Model file for the job. Use its own axes, mm. Coordinates: 2 decimals unless noted, no trailing zeros. Loops run counter-clockwise (first coordinate to the right, second up) from the corner with the lowest first, then second, coordinate; pieces in that order, holes last. Notation, with made-up numbers: M 79,45 L 100,45 A22 cw 100,76 Z; hole C -36,57.25 d11. An arc over 180 degrees is marked long. Write item = value, one per line. Start each with the question number.
from build123d import *

# Parameters (mm, degrees)
BOSS_EXTRUDE2_DEPTH      = 3
FILLET3_R                = 10
FILLET3_OF_MIRROR3_R     = 10
BOSS_EXTRUDE3_START      = -3
BOSS_EXTRUDE3_DEPTH      = 3
F_2_0_2_DIAMETER_HOLE1_D = 2


with BuildPart() as part:
    # Sketch2 → Boss-Extrude2 (new body)
    with BuildSketch(Plane(origin=(0, 0, 0), x_dir=(1, 0, 0), z_dir=(0, 1, 0))):
        with BuildLine():
            ThreePointArc((0, 117.185905081), (5, 117.120320028), (9.996559473, 116.923609999))
            ThreePointArc((9.996559473, 116.923609999), (7.163202874, 124.163621369), (0, 127.185905081))
            Line((0, 127.185905081), (0, 117.185905081))
        make_face()
        with BuildLine():
            Line((75, 92.603329386), (75, 4.814094919))
            ThreePointArc((75, 4.814094919), (82.067539985, 0.118365096), (86.763269807, 7.185905081))
            Line((86.763269807, 7.185905081), (85, 17.185905081))
            Line((85, 17.185905081), (85, 97.185905081))
            ThreePointArc((85, 97.185905081), (43.660622991, 112.118552795), (0, 117.185905081))
            Line((0, 117.185905081), (0, 109.185905081))
            ThreePointArc((0, 109.185905081), (38.343884954, 104.711356725), (75, 92.603329386))
        make_face()
    boss_extrude2 = extrude(amount=BOSS_EXTRUDE2_DEPTH)

    # Fillet3
    fillet3_edges = [part.edges().sort_by_distance(p)[0] for p in [
        (9.996559473, 1.5, -116.923609999),
        (85, 1.5, -97.185905081),
    ]]
    fillet(fillet3_edges, radius=FILLET3_R)

    # Mirror3: Boss-Extrude2 across plane
    add(boss_extrude2.mirror(Plane(origin=(0, 3, 0), x_dir=(0, 0, 1), z_dir=(1, 0, 0))))

    # Fillet3 of Mirror3
    fillet3_of_mirror3_edges = [part.edges().sort_by_distance(p)[0] for p in [
        (-9.996559473, 1.5, -116.923609999),
        (-85, 1.5, -97.185905081),
    ]]
    fillet(fillet3_of_mirror3_edges, radius=FILLET3_OF_MIRROR3_R)

    # Sketch4 → Boss-Extrude3 (add)
    with BuildSketch(Plane(origin=(0, 3, 0), x_dir=(1, 0, 0), z_dir=(0, 1, 0)).offset(BOSS_EXTRUDE3_START)):
        with BuildLine():
            Line((0, 109.185905081), (0, 106.185905081))
            ThreePointArc((0, 106.185905081), (2.927170094, 106.948379402), (5.110376179, 109.042013335))
            ThreePointArc((5.110376179, 109.042013335), (2.555670493, 109.131091975), (0, 109.185905081))
        make_face()
        with BuildLine():
            ThreePointArc((75, 92.603329386), (73.004956974, 93.481711721), (71, 94.337223109))
            ThreePointArc((71, 94.337223109), (72.171572875, 91.508795985), (75, 90.337223109))
            Line((75, 90.337223109), (75, 92.603329386))
        make_face()
        with BuildLine():
            Line((75, 73.103329386), (75, 82.103329386))
            ThreePointArc((75, 82.103329386), (70.5, 77.603329386), (75, 73.103329386))
        make_face()
    boss_extrude3 = extrude(amount=BOSS_EXTRUDE3_DEPTH)

    # Mirror4: Boss-Extrude3 across plane
    add(boss_extrude3.mirror(Plane(origin=(0, 0, 0), x_dir=(0, 0, 1), z_dir=(1, 0, 0))))

    # Ø2.0 (2) Diameter Hole1 (through all)
    with Locations(Plane(origin=(2.555188089, 3, -110.613959208), x_dir=(0, 0, 1), z_dir=(0, 1, 0))):
        with Locations((0, 0), (16.276736099, 72.444811911), (33.010629822, 72.444811911)):
            f_2_0_2_diameter_hole1 = Hole(F_2_0_2_DIAMETER_HOLE1_D / 2)

    # Mirror5: Ø2.0 (2) Diameter Hole1 across plane
    add(f_2_0_2_diameter_hole1.mirror(Plane(origin=(0, 0, 0), x_dir=(0, 0, 1), z_dir=(1, 0, 0))), mode=Mode.SUBTRACT)


solid = part.part
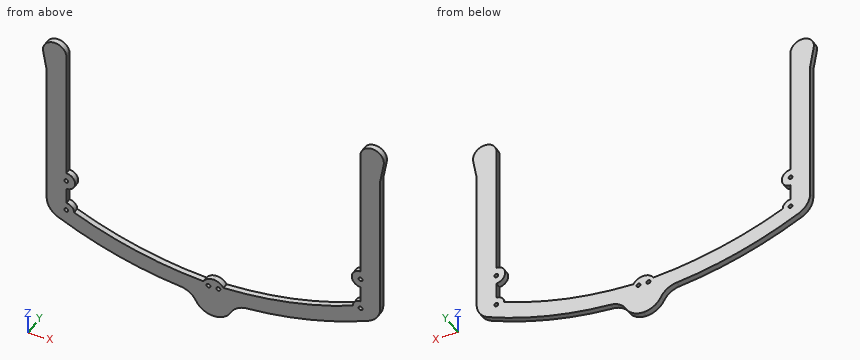
Item 1: Pin check, flat tips, straight feed: pin 1 Ø1.5 at (y, z) = (1, -85) entering from -X; pin 2 Ø1.5 at (y, z) = (1, -84.5) entering from +X; pin 3 Ø1.2 at (x, z) = (-75, -77.6) entering from +Y; pin 4 Ø1.5 at (x, y) = (-31.5, 2) entering from +Z. Stop position of each tip, or through.
Item 2: Cut at B-B (x = -62). Give the cut face in (y, z), plus the area to 3 significant figures.
Item 3: Cut at D-D (x = 36). Give the cut face in (y, z), plus the area to 3 significant figures.
Item 4: Probe L1, parallel to X at y = 0.95, z = -52; L2, parallel to X at y = 2.15, z = -5.5; L3, parallel to Z at x = 72.5, y = 0.2. List the from-to ranges inside material, lowest first.
Item 5: Cut at C-C (y = 2.25). Give the number of separate pieces and of enclosed holes in the cut face, plus the area to 3 significant figures.
Item 6: Cut at A-A (z = -66.5). Give the cut face in (x, y).
Reported:
q1.pin_1 = -85
q1.pin_2 = 85
q1.pin_3 = through
q1.pin_4 = -105.95
q2.outline = M 0,-106.82 L 3,-106.82 L 3,-97.85 L 0,-97.85 Z
q2.area = 26.9 mm^2
q3.outline = M 0,-113.76 L 3,-113.76 L 3,-105.21 L 0,-105.21 Z
q3.area = 25.6 mm^2
q4.L1 = -85 to -75, 75 to 85
q4.L2 = -86.86 to -75, 75 to 86.86
q4.L3 = -102.86 to -91.21, -81.34 to -73.86
q5.separate_pieces = 1
q5.enclosed_holes = 6
q5.area = 3,540 mm^2
q6.outline = M -85,0 L -75,0 L -75,3 L -85,3 Z; M 75,0 L 85,0 L 85,3 L 75,3 Z
